Job drawing, mm, ordinate dimensions from the low corner. One solid piece. Give positions to 0.01 mm unless a question says otherwise; leave off trailing zeros. Loops run counter-clockwise (first coordinate to the right, second up) from the corner with the lowest first, then second, coordinate; pieces in that order, holes last. Notation, with made-up numbers: M 31.5,42 L 57.5,42 A15 cw 57.5,59 Z; hole C 1.5,-18 d4. An arc over 180 degrees is marked long. Put each result on its own line as item: value.
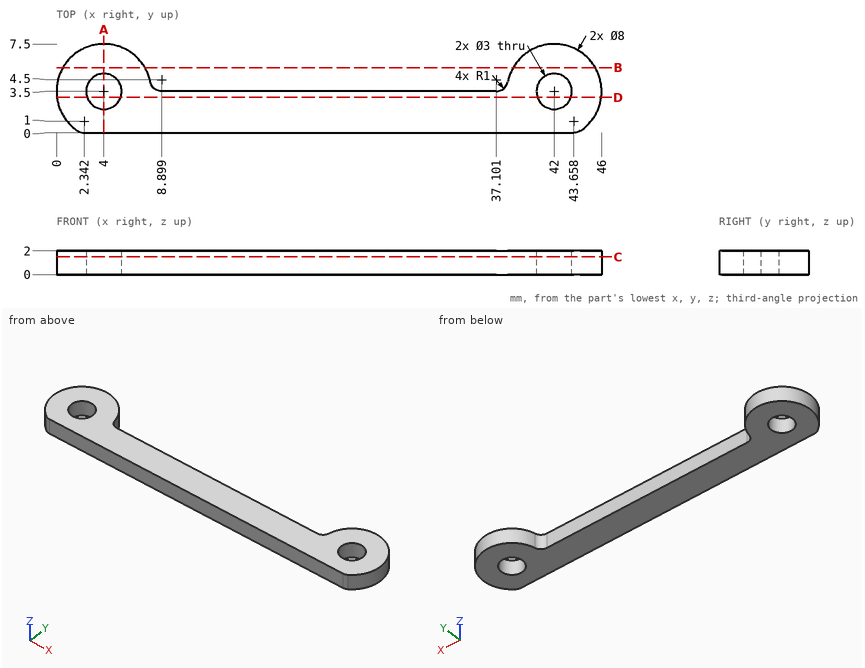
Q1. Slice it at B-B (y = 5.5). List the corners of the cut face in (x, z), and give its area (3 significant figures).
Here are the results:
outline: M 0.54,0 L 7.46,0 L 7.46,2 L 0.54,2 Z; M 38.54,0 L 45.46,0 L 45.46,2 L 38.54,2 Z
area: 27.7 mm²
Q2. Drop flat-ended pins along their axis: pin 1 Ø2.5 at (x, y) = (4, 3.5) entering from -Z; pin 2 Ø0.6 at (x, z) = (26, 1) entering from +Y; pin 3 Ø1 at (y, z) = (2, 0.5) entering from -X. Give the stop position or say it passes through.
Here are the results:
pin 1: through
pin 2: y = 3.5
pin 3: x = 0.13
Q3. Slice it at A-A (x = 4). List the corners of the cut face in (y, z).
Here are the results:
outline: M 0,0 L 2,0 L 2,2 L 0,2 Z; M 5,0 L 7.5,0 L 7.5,2 L 5,2 Z
Q4. Slice it at D-D (y = 3). List the corners of the cut face in (x, z).
Here are the results:
outline: M 0.03,0 L 2.59,0 L 2.59,2 L 0.03,2 Z; M 5.41,0 L 40.59,0 L 40.59,2 L 5.41,2 Z; M 43.41,0 L 45.97,0 L 45.97,2 L 43.41,2 Z
Q5. Probe line 1 (Y direction, x = 42, z = 0.45); line 2 (X direction, y = 2.5, z = 0.15); line 3 (X direction, y = 6.75, z = 1). List the from-to ranges inside material, lowest first. Write a range as from..to.
Here are the results:
line 1: 0..2, 5..7.5
line 2: 0.13..2.88, 5.12..40.88, 43.12..45.87
line 3: 1.67..6.33, 39.67..44.33
Q6. Slice it at C-C (z = 1.5). List the corners of the cut face in (x, y), and give its area (3 significant figures).
Here are the results:
outline: M 1.79,0.17 A1 ccw 2.34,0 L 43.66,0 A1 ccw 44.21,0.17 A4 ccw long 38.08,4.3 A1 cw 37.1,3.5 L 8.9,3.5 A1 cw 7.92,4.3 A4 ccw long Z; hole C 4,3.5 d3; hole C 42,3.5 d3
area: 193 mm²
